from build123d import *

# Parameters (mm, degrees)
F0_R     = 5
F1_DEPTH = 15
F3_R     = 1.5
F3_R_2   = 1
F4_DEPTH = 26


# Not quite as in the source:
# - a feature names something its author has since deleted; it is built from what else it names


with BuildPart() as f1:
    # F0 (on Top) → F1 (new body)
    with BuildSketch(Plane.XY):
        Polygon((-37.5, 9.6315789474), (-37.5, -5.3684210526), (37.5, -5.3684210526), (37.5, 9.6315789474), (20, 9.6315789474), (20, 14.2315789474), (-20, 14.2315789474), (-20, 9.6315789474), align=None)
        with Locations((-29.8843569823, 2.6315789474)):
            Circle(F0_R, mode=Mode.SUBTRACT)
        with Locations((29.8843569823, 2.6315789474)):
            Circle(F0_R, mode=Mode.SUBTRACT)
    extrude(amount=F1_DEPTH)

    # F3 (on offset) → F4 (join, symmetric)
    with BuildSketch(Plane(origin=(0, 0, 0), x_dir=(0, -1, 0), z_dir=(-1, 0, 0))):
        with Locations((-15.7305789474, 1)):
            Circle(F3_R)
        with Locations((-15.7305789474, 1)):
            Circle(F3_R_2, mode=Mode.SUBTRACT)
    extrude(amount=F4_DEPTH, both=True)


solid = f1.part
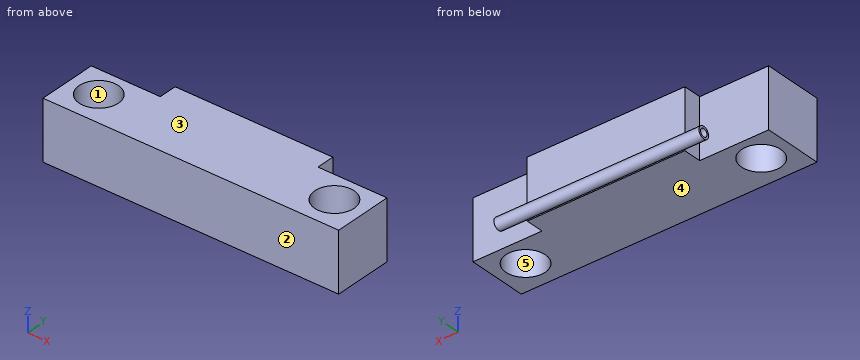
The listing builds one solid part. Answer for the finished solid, in the listing's coordinates (mm). Face numbers are marked on the shaded views. A direction names the side the tool comes from. Give positions to 0.01 mm unless a question says otherwise; leave off trailing zeros. Write each loop counter-clockwise with the first axis right and the second up, starting at its lowest first coordinate (ties: lowest second). Pieces come first, ordered by that corner, then holes.
Item 1: Which of the six approach directions +Z, -Z, +X, -X, +Y, -Y give full straight-line access (tool end or side, diameter ignored) to the marked faces 4 and 5?
Item 2: Section C-C, the plane x = -6.5 is taken. Write down the section's boundary in (y, z).
Item 3: Section A-A, the plane x = 22 is taken. Write down the section's boundary in (y, z), plus the area to 3 significant figures.
Item 4: Find the intervals of material crossed by line 1 along X through (y, z) = (2.75, 11.75); line 2 along X through (y, z) = (-0.5, 12); line 3 along Y through (x, z) = (20.5, 3.75), in increasing order.
Item 5: Flat-ended cylindrical pins translate along their axes: P1, Ø6, axis at x = 8.5, y = 4, coming from the -Z side; P2, Ø4, axis at y = 14, z = 9, coming from the +X side; P3, Ø1, axis at x = 2.5, z = 0.5, coming from the +Y side; P4, Ø2, axis at y = 13.5, z = 2.5, coming from the -X side. Find the tip coordinate at first contact, or state that the pin passes through.
Item 6: Section D-D, the plane z = 11 is taken. Write down the section's boundary in (x, y).
Item 7: Section B-B, the plane y = 5.25 is taken. Write down the section's boundary in (x, z), plus the area to 3 significant figures.
Item 8: Determine the mould class of the marked faces 1, 2 and 3 for opening direction Y: released by +Y, released by -Y, zero draft, split by the parting line, or undercut.
Completed:
1. face 4: -Z, +X, -X, -Y
1. face 5: +Z, -Z
2. outline: (-5.37, 0) - (14.23, 0) - (14.23, 0.95) arc R1.5 ccw (long way) to (14.23, 1.05) - (14.23, 15) - (-5.37, 15) - close; hole circle Ø2 at (15.73, 1)
3. outline: (-5.37, 0) - (9.63, 0) - (9.63, 15) - (-5.37, 15) - close; circle Ø3 at (15.73, 1); hole circle Ø2 at (15.73, 1)
3. area: 229 mm2
4. line 1: x = -37.5 to -34.88, -24.89 to 24.89, 34.88 to 37.5
4. line 2: x = -37.5 to -33.78, -25.99 to 25.99, 33.78 to 37.5
4. line 3: y = -5.37 to 9.63
5. P1: stops at z = 0
5. P2: stops at x = 20
5. P3: stops at y = 17.23
5. P4: stops at x = -20
6. outline: (-37.5, -5.37) - (37.5, -5.37) - (37.5, 9.63) - (20, 9.63) - (20, 14.23) - (-20, 14.23) - (-20, 9.63) - (-37.5, 9.63) - close; hole circle Ø10 at (-29.88, 2.63); hole circle Ø10 at (29.88, 2.63)
7. outline: (-37.5, 0) - (-34.14, 0) - (-34.14, 15) - (-37.5, 15) - close; (-25.62, 0) - (25.62, 0) - (25.62, 15) - (-25.62, 15) - close; (34.14, 0) - (37.5, 0) - (37.5, 15) - (34.14, 15) - close
7. area: 869 mm2
8. face 1: undercut
8. face 2: released by -Y
8. face 3: zero draft
